For this review, use the dimensioned drawing (mm, ordinates from the lowest corner) and the shaded views. A direction names the side the tool comes from. Coordinates: 2 decimals unless noted, no trailing zeros. Loops run counter-clockwise (first coordinate to the right, second up) from the corner with the lowest first, then second, coordinate; pieces in that order, holes last. Notation, with made-up numbers: (23.5, 11.5) -> (62.5, 11.5) arc R19 ccw to (62.5, 42.5) -> close; hole circle Ø5 at (-30, 19.25). An arc over 180 degrees is marked (long way). Answer as a JSON object with one key per item and string values.
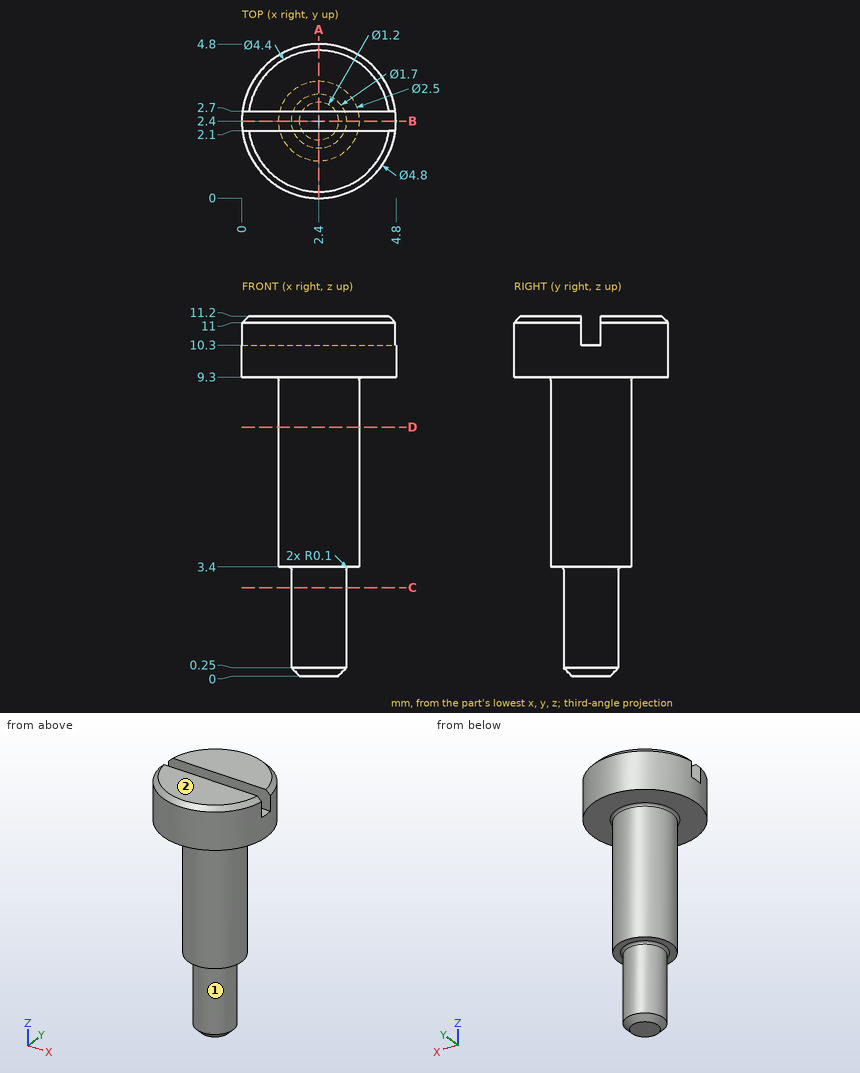
1) Add section D-D, the plane z = 7.75. Give the boundary of the cut face in (x, y), and give its area (3 significant figures).
Completed:
{"outline": "circle Ø2.5 at (2.4, 2.4)", "area": "4.91 mm²"}
2) Add section C-C, the plane z = 2.75. Give the boundary of the cut face in (x, y), and give its area (3 significant figures).
Completed:
{"outline": "circle Ø1.7 at (2.4, 2.4)", "area": "2.27 mm²"}
3) For the marked faces 1 and 2, list the 3-axis set-ups (+Z, -Z, +X, -X, +Y, -Y) from which the entire face can be reached by the end or side of a thin tool; tool diameter is ignored.
Completed:
{"face 1": "-Z", "face 2": "+Z, +X, -X, +Y, -Y"}
4) Add section B-B, the plane y = 2.4. Give the boundary of the cut face in (x, z), and give its area (3 significant figures).
Completed:
{"outline": "(0, 9.3) -> (1.05, 9.3) arc R0.1 cw to (1.15, 9.2) -> (1.15, 3.4) -> (1.45, 3.4) arc R0.1 cw to (1.55, 3.3) -> (1.55, 0.25) -> (1.8, 0) -> (3, 0) -> (3.25, 0.25) -> (3.25, 3.3) arc R0.1 cw to (3.35, 3.4) -> (3.65, 3.4) -> (3.65, 9.2) arc R0.1 cw to (3.75, 9.3) -> (4.8, 9.3) -> (4.8, 10.3) -> (0, 10.3) -> close", "area": "25.3 mm²"}
5) Add section A-A, the plane x = 2.4. Give the boundary of the cut face in (y, z), and give its area (3 significant figures).
Completed:
{"outline": "(0, 9.3) -> (1.05, 9.3) arc R0.1 cw to (1.15, 9.2) -> (1.15, 3.4) -> (1.45, 3.4) arc R0.1 cw to (1.55, 3.3) -> (1.55, 0.25) -> (1.8, 0) -> (3, 0) -> (3.25, 0.25) -> (3.25, 3.3) arc R0.1 cw to (3.35, 3.4) -> (3.65, 3.4) -> (3.65, 9.2) arc R0.1 cw to (3.75, 9.3) -> (4.8, 9.3) -> (4.8, 11) -> (4.6, 11.2) -> (2.7, 11.2) -> (2.7, 10.3) -> (2.1, 10.3) -> (2.1, 11.2) -> (0.2, 11.2) -> (0, 11) -> close", "area": "29.0 mm²"}
6) Wall thickness on probe 1 along Z at (x, y) = (4.1, 2.35); probe 2 along X at (y, z) = (1.8, 1.25); probe 3 along Z at (x, y) = (1.5, 3.4): over which ranges is each line inside the solid? List them lowest first.
Completed:
{"probe 1": "9.3 to 10.3", "probe 2": "1.8 to 3", "probe 3": "9.3 to 11.2"}
7) Clearance check with flat-ended pins moving along their axes: pin 1 Ø1.5 at (x, z) = (3, 7.5) entering from +Y; pin 2 Ø1 at (x, z) = (3.5, 5) entering from -Y. State where each tip first meets the part, or that it passes through.
Completed:
{"pin 1": "y = 3.65", "pin 2": "y = 1.3"}
